For this review, take the finished solid that the model builds, in its own axes (mm). Coordinates: 2 decimals unless noted, no trailing zeros. Loops run counter-clockwise (first coordinate to the right, second up) from the corner with the lowest first, then second, coordinate; pieces in that order, holes last.
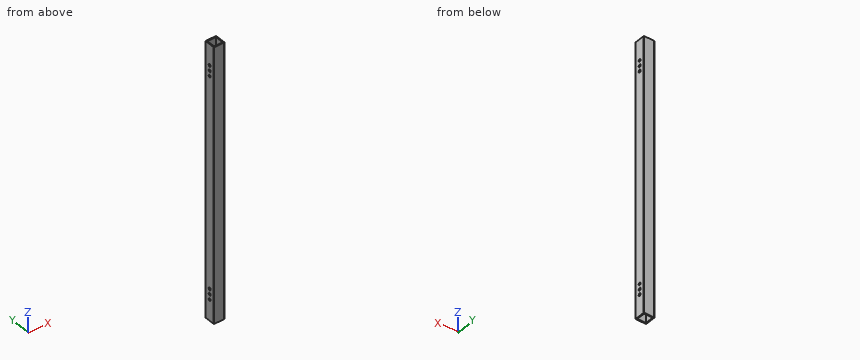
```python
from build123d import *

# Parameters (mm, degrees)
F0_W     = 25.4
F0_H     = 25.4
F0_W_2   = 20.32
F0_H_2   = 20.32
F1_DEPTH = 660.4
F4_D     = 6.35
F5_R     = 0.762


with BuildPart() as f1:
    # F0 (on Top) → F1 (new body)
    with BuildSketch(Plane.XY):
        Rectangle(F0_W, F0_H)
        Rectangle(F0_W_2, F0_H_2, mode=Mode.SUBTRACT)
    extrude(amount=F1_DEPTH)

    # F4 (through all)
    with Locations(Plane.YZ.offset(12.7)):
        with Locations((0, 609.6), (0, 596.9), (0, 584.2), (0, 76.2), (0, 63.5), (0, 50.8)):
            Hole(F4_D / 2)

    # F5
    f5_edges = [f1.edges().sort_by_distance(p)[0] for p in [
        (12.7, 12.7, 330.2),
        (-12.7, 12.7, 330.2),
        (12.7, -12.7, 330.2),
        (-12.7, -12.7, 330.2),
    ]]
    fillet(f5_edges, radius=F5_R)


solid = f1.part
```
Q1. Consider section B-B (z = 121). State the section outline as (x, y) points.
Q2. Wall thickness on probe 1 along Y at (x, z) = (9, 273); probe 2 along Y at (x, z) = (11.7, 584.2) (3 decimals): over which ranges is each line inside the solid? List them lowest first.
Q3. For pin 1 Ø7.5 at (y, z) = (0, 596.9) entering from +X; pin 2 Ø5 at (y, z) = (0, 63.5) entering from -X, all flat-tipped, find the tip position at first contact; note any pin that passes through.
Q4. Consider section A-A (x = -5.75). State the section outline as (y, z) points, then the cut area to 3 significant figures.
Model answer:
1. outline: (-12.7, -11.94) arc R0.76 ccw to (-11.94, -12.7) - (11.94, -12.7) arc R0.76 ccw to (12.7, -11.94) - (12.7, 11.94) arc R0.76 ccw to (11.94, 12.7) - (-11.94, 12.7) arc R0.76 ccw to (-12.7, 11.94) - close; hole (-10.16, -10.16) - (10.16, -10.16) - (10.16, 10.16) - (-10.16, 10.16) - close
2. probe 1: y = -12.7 to -10.16, 10.16 to 12.7
2. probe 2: y = -12.7 to -3.175, 3.175 to 12.7
3. pin 1: stops at x = 12.7
3. pin 2: passes through
4. outline: (-12.7, 0) - (-10.16, 0) - (-10.16, 660.4) - (-12.7, 660.4) - close; (10.16, 0) - (12.7, 0) - (12.7, 660.4) - (10.16, 660.4) - close
4. area: 3,350 mm2
